```python
from build123d import *

# Parameters (mm, degrees)
EXTRUDE_1_DEPTH     = 45
CUT_EXTRUDE_START   = -20.5
CUT_EXTRUDE_1_DEPTH = 20.5
FILLET_1_R          = 1.8


with BuildPart() as part:
    # 草图2 → 凸台-拉伸1 (new body)
    with BuildSketch(Plane.XY):
        with BuildLine():
            Line((-17.000000000000004, 25.99999999999999), (-6.324555320336758, 25.999999999999996))
            ThreePointArc((-6.324555320336758, 25.999999999999996), (-4.720987868862212, 26.464537235814447), (-3.614031611621006, 27.71428571428571))
            ThreePointArc((-3.614031611621006, 27.71428571428571), (2.4e-16, 30), (3.614031611621006, 27.71428571428571))
            ThreePointArc((3.614031611621006, 27.71428571428571), (4.720987868862212, 26.464537235814447), (6.324555320336758, 25.999999999999996))
            Line((6.324555320336758, 25.999999999999996), (17.000000000000004, 25.99999999999999))
            ThreePointArc((17.000000000000004, 25.99999999999999), (33.14520180681835, 20.379707029717306), (42.310344827586206, 5.948650662854563))
            ThreePointArc((42.310344827586206, 5.948650662854563), (43.01263196777571, 4.615165346220191), (44.27472527472528, 3.7914476752259816))
            ThreePointArc((44.27472527472528, 3.7914476752259816), (47, -7.66e-15), (44.27472527472528, -3.791447675225999))
            ThreePointArc((44.27472527472528, -3.791447675225999), (43.01263196777571, -4.615165346220208), (42.310344827586206, -5.948650662854578))
            ThreePointArc((42.310344827586206, -5.948650662854578), (38.72710851162517, -14.280502642556568), (32.5, -20.874625745148098))
            Line((32.5, -20.874625745148098), (30.413461538461537, -18.064579971762782))
            ThreePointArc((30.413461538461537, -18.064579971762782), (38.36238574416096, 7.063885284860494), (17.000000000000007, 22.500000000000004))
            Line((17.000000000000007, 22.500000000000004), (1.9364916731037032, 22.499999999999996))
            ThreePointArc((1.9364916731037032, 22.499999999999996), (2.4e-16, 22), (-1.9364916731037032, 22.499999999999996))
            Line((-1.9364916731037032, 22.499999999999996), (-17.000000000000004, 22.500000000000004))
            ThreePointArc((-17.000000000000004, 22.500000000000004), (-38.36238574416096, 7.063885284860502), (-30.413461538461544, -18.064579971762775))
            Line((-30.413461538461544, -18.064579971762775), (-32.5, -20.874625745148098))
            ThreePointArc((-32.5, -20.874625745148098), (-38.727108511625175, -14.280502642556563), (-42.310344827586206, -5.948650662854575))
            ThreePointArc((-42.310344827586206, -5.948650662854575), (-43.01263196777571, -4.615165346220205), (-44.27472527472528, -3.7914476752259954))
            ThreePointArc((-44.27472527472528, -3.7914476752259954), (-46.99999999999999, -3.62e-15), (-44.27472527472527, 3.791447675225978))
            ThreePointArc((-44.27472527472527, 3.791447675225978), (-43.012631967775704, 4.615165346220189), (-42.310344827586206, 5.9486506628545595))
            ThreePointArc((-42.310344827586206, 5.9486506628545595), (-33.14520180681835, 20.379707029717306), (-17.000000000000004, 25.99999999999999))
        make_face()
        Polygon((1.414508159514589, 28.45), (-1.4145081595145819, 28.45), (-2.829016319029165, 26.000000000000004), (-1.4145081595145819, 23.549999999999997), (1.4145081595145816, 23.549999999999997), (2.829016319029169, 26.000000000000004), align=None, mode=Mode.SUBTRACT)
        Polygon((-43, -2.8290163190291664), (-45.44999999999999, -1.414508159514586), (-45.44999999999999, 1.4145081595145663), (-43, 2.8290163190291495), (-40.55, 1.4145081595145712), (-40.55, -1.414508159514584), align=None, mode=Mode.SUBTRACT)
        Polygon((45.44999999999999, -1.414508159514587), (45.44999999999999, 1.4145081595145672), (43, 2.8290163190291513), (40.55, 1.414508159514572), (40.55, -1.414508159514585), (43, -2.829016319029168), align=None, mode=Mode.SUBTRACT)
    extrude(amount=EXTRUDE_1_DEPTH)

    # 草图3 → 切除-拉伸1 (cut)
    with BuildSketch(Plane.XY.offset(45).offset(CUT_EXTRUDE_START)):
        with BuildLine():
            Line((-42.16101815897212, 6.551577306563255), (-38.773958022187415, 5.669634207602821))
            ThreePointArc((-38.773958022187415, 5.669634207602821), (-30.76014589909817, 17.801920818707508), (-17.000000000000004, 22.5))
            Line((-17.000000000000004, 22.5), (-6.499999999999999, 22.5))
            Line((-6.499999999999999, 22.5), (-6.500000000000001, 25.999999999999986))
            Line((-6.500000000000001, 25.999999999999986), (-17.000000000000004, 25.999999999999993))
            ThreePointArc((-17.000000000000004, 25.999999999999993), (-32.900613038957886, 20.57110850161755), (-42.16101815897212, 6.551577306563255))
        make_face()
        with BuildLine():
            Line((42.16101815897216, 6.551577306563108), (38.77395802218746, 5.669634207602693))
            ThreePointArc((38.77395802218746, 5.669634207602693), (30.760145899098227, 17.80192081870747), (17.000000000000007, 22.5))
            Line((17.000000000000007, 22.5), (6.500000000000001, 22.5))
            Line((6.500000000000001, 22.5), (6.500000000000003, 25.999999999999986))
            Line((6.500000000000003, 25.999999999999986), (17, 25.99999999999999))
            ThreePointArc((17, 25.99999999999999), (32.90061303895794, 20.57110850161751), (42.16101815897216, 6.551577306563108))
        make_face()
    extrude(amount=CUT_EXTRUDE_1_DEPTH, mode=Mode.SUBTRACT)

    # 圆角1
    # the kernel refuses this fillet: 1.8 mm, written as the material it takes off along each edge
    with BuildSketch(Plane(origin=(-6.499999999999999, 22.5, 24.5), x_dir=(-4.9e-16, 1, 0), z_dir=(0, 0, 1))) as fillet_1_piece_1:
        with BuildLine():
            CenterArc((FILLET_1_R, -FILLET_1_R), FILLET_1_R, 89.99999999999997, 89.99999999999997)
            Line((-4.44e-15, -FILLET_1_R), (0, 0))
            Line((0, 0), (FILLET_1_R, 0))
        make_face()
    extrude(amount=25, mode=Mode.SUBTRACT)
    with BuildSketch(Plane(origin=(-6.500000000000001, 25.999999999999986, 24.5), x_dir=(0.9891271990467642, 0.14706251767837725, 0), z_dir=(0, 0, 1))) as fillet_1_piece_2:
        with BuildLine():
            CenterArc((1.5573753123133534, -1.7649481565014509), FILLET_1_R, 101.3256751198377, 70.21759155918191)
            Line((-0.22305364597082192, -1.5002356246803719), (-0.4010965417992392, -1.473764371498264))
            Line((-0.4010965417992392, -1.473764371498264), (-0.17804289582841726, 0.02647125318210786))
            Line((-0.17804289582841726, 0.02647125318210786), (0.02647125318210786, 0.17804289582841726))
            ThreePointArc((0.02647125318210786, 0.17804289582841726), (0.2000083577650695, 0.15224155952387494), (1.168531917251559, 0.17649481565014538))
            Line((1.168531917251559, 0.17649481565014538), (1.203881316802631, -2e-17))
        make_face()
    extrude(amount=24.291816730260194, mode=Mode.SUBTRACT)
    with BuildSketch(Plane(origin=(6.500000000000001, 22.5, 24.5), x_dir=(-1, -1.97e-15, 0), z_dir=(0, 0, 1))) as fillet_1_piece_3:
        with BuildLine():
            CenterArc((FILLET_1_R, -FILLET_1_R), FILLET_1_R, 89.99999999999993, 89.99999999999996)
            Line((-4.44e-15, -FILLET_1_R), (0, 0))
            Line((0, 0), (FILLET_1_R, 0))
        make_face()
    extrude(amount=25, mode=Mode.SUBTRACT)
    with BuildSketch(Plane(origin=(6.500000000000003, 25.999999999999986, 24.5), x_dir=(-0.9891271990467642, 0.14706251767837714, 0), z_dir=(0, 0, 1))) as fillet_1_piece_4:
        with BuildLine():
            CenterArc((1.5573753123133545, 1.7649481565014509), FILLET_1_R, 188.4567333209804, 70.21759155918187)
            Line((-0.22305364597082086, 1.5002356246803719), (-0.40109654179923815, 1.4737643714982642))
            Line((-0.40109654179923815, 1.4737643714982642), (-0.17804289582841726, -0.02647125318210784))
            Line((-0.17804289582841726, -0.02647125318210784), (0.02647125318210784, -0.17804289582841726))
            ThreePointArc((0.02647125318210784, -0.17804289582841726), (0.20000835776506773, -0.15224155952387522), (1.1685319172515596, -0.17649481565014538))
            Line((1.1685319172515596, -0.17649481565014538), (1.2038813168026317, 2e-17))
        make_face()
    extrude(amount=24.291816730260194, mode=Mode.SUBTRACT)
    with BuildSketch(Plane(origin=(38.77395802218746, 5.669634207602693, 24.5), x_dir=(0.2159440686633983, -0.9764057349325113, 0), z_dir=(0, 0, 1))) as fillet_1_piece_5:
        with BuildLine():
            CenterArc((1.7345250396355076, 1.7987633090933175), FILLET_1_R, 182.12401133336417, 85.75197733327184)
            Line((-0.06423826945781225, 1.7320508075688776), (0, 0))
            ThreePointArc((0, 0), (0.8339062690555353, 0.01545863633349137), (1.6678125381110727, -6e-17))
        make_face()
    extrude(amount=24.83310408026317, mode=Mode.SUBTRACT)
    with BuildSketch(Plane(origin=(42.16101815897217, 6.551577306563109, 24.5), x_dir=(0.30232503982893916, -0.9532048941819542, 0), z_dir=(0, 0, 1))) as fillet_1_piece_6:
        with BuildLine():
            CenterArc((1.7095969183976014, -1.770799573138055), FILLET_1_R, 100.33438988529196, 76.6632370150231)
            Line((-0.08793234080970554, -1.6765204010286838), (-0.267685266730436, -1.667092483817746))
            Line((-0.267685266730436, -1.667092483817746), (-0.17975292592072528, 0.00942791721106288))
            Line((-0.17975292592072528, 0.00942791721106288), (0.00942791721106515, 0.17975292592072362))
            ThreePointArc((0.00942791721106515, 0.17975292592072362), (0.633577059222906, 0.1395355017085772), (1.3543993186778904, 0.1770799573138067))
            Line((1.3543993186778904, 0.1770799573138067), (1.3866900095614998, -3e-17))
        make_face()
    extrude(amount=24.697062031666952, mode=Mode.SUBTRACT)
    with BuildSketch(Plane(origin=(-38.773958022187415, 5.669634207602822, 24.5), x_dir=(-0.21594406866341104, -0.9764057349325085, 0), z_dir=(0, 0, 1))) as fillet_1_piece_7:
        with BuildLine():
            CenterArc((1.7345250396355227, -1.7987633090933188), FILLET_1_R, 92.12401133336449, 85.75197733327163)
            Line((-0.06423826945779765, -1.7320508075688876), (0, 0))
            ThreePointArc((0, 0), (0.8339062690555384, -0.01545863633350171), (1.6678125381110729, 3e-17))
        make_face()
    extrude(amount=24.833104080263197, mode=Mode.SUBTRACT)
    with BuildSketch(Plane(origin=(-42.16101815897213, 6.5515773065632565, 24.5), x_dir=(-0.30232503982891934, -0.9532048941819604, 0), z_dir=(0, 0, 1))) as fillet_1_piece_8:
        with BuildLine():
            CenterArc((1.7095969183976452, 1.770799573138059), FILLET_1_R, 183.00237309968935, 76.66323701501943)
            Line((-0.08793234080965445, 1.676520401028549), (-0.26768526673038506, 1.6670924838176002))
            Line((-0.26768526673038506, 1.6670924838176002), (-0.17975292592072462, -0.00942791721105888))
            Line((-0.17975292592072462, -0.00942791721105888), (0.00942791721106057, -0.1797529259207241))
            ThreePointArc((0.00942791721106057, -0.1797529259207241), (0.6335770592230675, -0.13953550170858298), (1.3543993186779588, -0.1770799573138045))
            Line((1.3543993186779588, -0.1770799573138045), (1.3866900095615668, 2e-17))
        make_face()
    extrude(amount=24.697062031666604, mode=Mode.SUBTRACT)


solid = part.part
```
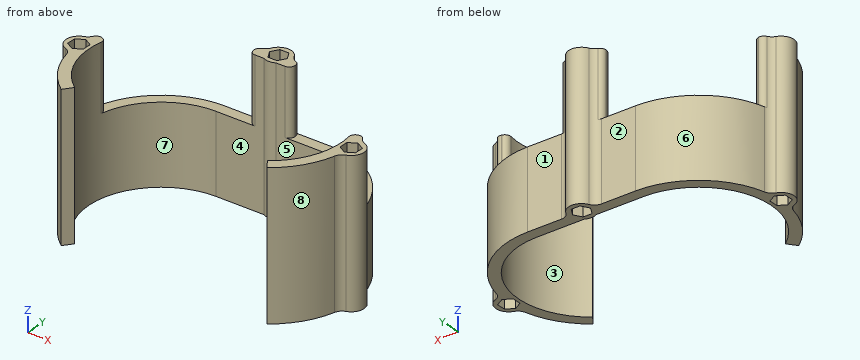
The listing builds one solid part. Answer for the finished solid, in the listing's coordinates (mm). Face numbers are marked on the shaded views. A direction names the side the tool comes from. Coordinates: 2 decimals unless noted, no trailing zeros. Loops run counter-clockwise (first coordinate to the right, second up) from the corner with the lowest first, then second, coordinate; pieces in that order, holes last. Notation, with made-up numbers: M -12,-38 L 36,-38 A6 ccw 36,-30 Z; hole C -12,33.25 d9. An arc over 180 degrees is marked long. Answer as a JSON object with one key per item and string values. Group by question number.
Item 1: Which of the six approach directions +Z, -Z, +X, -X, +Y, -Y give full straight-line access (tool end or side, diameter ignored) to the marked faces 1, 2, 3 and 4?
Item 2: Consider L1, parallel to X at y = 1, z = 40.5; L2, parallel to Y at x = -6.5, z = 2; L3, parallel to X at y = 12, z = 23. Determine where each line is inside the solid, lowest interval first.
Item 3: Determine the mould class of the marked faces 5, 6, 7 and 8 for opening direction X: +X half, -X half, draft (parallel to the pull), parting line (faces both ways), or undercut.
Item 4: Section A-A (y = 15) is taken. Write down the section's boundary in (x, z).
Item 5: Each of these flat-tipped pins is pushed along its axis until it touches: P1, Ø4.5, axis at x = -11, z = 17, coming from the -Y side; P2, Ø6.5, axis at x = -29.5, y = 18.5, coming from the +Z side; P3, Ø2, axis at y = -6, z = 19, coming from the +X side; P4, Ø8, axis at x = 33, y = 9, coming from the -Z side. Where does it stop, or does it pass through?
Item 6: Section B-B (x = 36) is taken. Write down the section's boundary in (y, z).
Item 7: Section C-C (z = 30) is taken. Give the number of separate pieces and of enclosed holes in the cut face, and give its area (3 significant figures).
Solved:
{
 "1": {"face 1": "+Z, -Z, +X, +Y", "face 2": "+Z, -Z, -X, +Y", "face 3": "+Z, -Z", "face 4": "+Z, -Z, -Y"},
 "2": {"L1": "x = -46.87 to -45.45, -40.55 to -39.48, 39.48 to 40.55, 45.45 to 46.87", "L2": "y = 22.5 to 26", "L3": "x = -40.07 to -36.03, 36.03 to 40.07"},
 "3": {"face 5": "undercut", "face 6": "-X half", "face 7": "undercut", "face 8": "+X half"},
 "4": {"outline": "M -38.24,0 L -33.77,0 L -33.77,24.5 L -38.24,24.5 Z; M 33.77,0 L 38.24,0 L 38.24,24.5 L 33.77,24.5 Z"},
 "5": {"P1": "stops at y = 22.5", "P2": "stops at z = 24.5", "P3": "stops at x = 42.72", "P4": "passes through"},
 "6": {"outline": "M -17.75,0 L -12.05,0 L -12.05,45 L -17.75,45 Z; M 12.05,0 L 17.75,0 L 17.75,24.5 L 12.05,24.5 Z"},
 "7": {"separate pieces": "3", "enclosed holes": "3", "area": "263 mm2"}
}
